Here's how the part is built. I have some questions about the finished solid (model axes, mm). Give positions to 0.01 mm unless a question says otherwise; leave off trailing zeros. Loops run counter-clockwise (first coordinate to the right, second up) from the corner with the lowest first, then second, coordinate; pieces in that order, holes last.
Q1. Suppose I cut it at B-B (x = 0). List the corners of the cut face in (y, z) for me, and give its area (3 significant figures).
Q2. I need wall thicknesses on probe 1 along X at (y, z) = (1.1, 0); probe 2 along Z at (x, y) = (0, 1.65); probe 3 along Z at (x, y) = (0, 0.8). Which ranges of each line are inside material? Lowest first, please.
Q3. I'm going to push a flat-ended pin straight in: P1, Ø3, axis at x = -1, z = 0.5, coming from the -Y side. Where does the tip first touch, or does it pass through?
Q4. Suppose I cut it at A-A (z = 0). List the corners of the cut face in (x, y) for me, and give its area (4 significant figures).
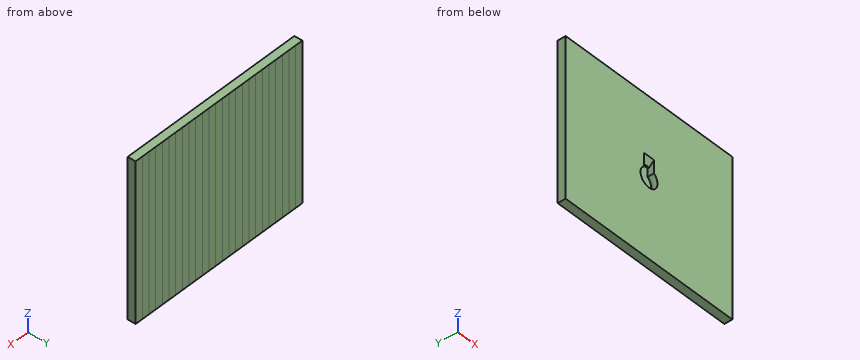
```python
from build123d import *

# Parameters (mm, degrees)
SKETCH1_W           = 59
SKETCH1_H           = 49.5
SKETCH1_R           = 3
BOSS_EXTRUDE1_DEPTH = 1.5
BOSS_EXTRUDE2_DEPTH = 49.5
CUT_EXTRUDE1_DEPTH  = 2
CUT_EXTRUDE3_DEPTH  = 65.105869466
CHAMFER3_SIZE       = 1.5
SKETCH7_W           = 59
SKETCH7_H           = 2.086537977
CUT_EXTRUDE5_DEPTH  = 58.762444547


with BuildPart() as part:
    # Sketch1 → Boss-Extrude1 (new body)
    with BuildSketch(Plane(origin=(0, 0, 0), x_dir=(1, 0, 0), z_dir=(0, 1, 0))):
        Rectangle(SKETCH1_W, SKETCH1_H)
        with Locations(Location((0, 0, 0), (0, 0, 270))):
            Circle(SKETCH1_R, mode=Mode.SUBTRACT)
    extrude(amount=BOSS_EXTRUDE1_DEPTH)

    # Sketch2 → Boss-Extrude2 (add)
    with BuildSketch(Plane(origin=(0, 0, -24.75), x_dir=(-1, 0, 0), z_dir=(0, 0, -1))):
        Polygon((-29.5, 1.5), (29.5, 1.5), (29.5, 2.5), (28.32, 4), (27.14, 2.5), (25.96, 4), (24.78, 2.5), (23.6, 4), (22.42, 2.5), (21.24, 4), (20.06, 2.5), (18.88, 4), (17.7, 2.5), (16.52, 4), (15.34, 2.5), (14.16, 4), (12.98, 2.5), (11.8, 4), (10.62, 2.5), (9.44, 4), (8.26, 2.5), (7.08, 4), (5.9, 2.5), (4.72, 4), (3.54, 2.5), (2.36, 4), (1.18, 2.5), (0, 4), (-1.18, 2.5), (-2.36, 4), (-3.54, 2.5), (-4.72, 4), (-5.9, 2.5), (-7.08, 4), (-8.26, 2.5), (-9.44, 4), (-10.62, 2.5), (-11.8, 4), (-12.98, 2.5), (-14.16, 4), (-15.34, 2.5), (-16.52, 4), (-17.7, 2.5), (-18.88, 4), (-20.06, 2.5), (-21.24, 4), (-22.42, 2.5), (-23.6, 4), (-24.78, 2.5), (-25.96, 4), (-27.14, 2.5), (-28.32, 4), (-29.5, 2.5), align=None)
    extrude(amount=-BOSS_EXTRUDE2_DEPTH)

    # Sketch3 → Cut-Extrude1 (cut)
    with BuildSketch(Plane(origin=(0, 0, 0), x_dir=(-1, 0, 0), z_dir=(0, -1, 0))):
        with BuildLine():
            Line((-1.75, -2.436698586), (-1.75, -5))
            Line((-1.75, -5), (1.75, -5))
            Line((1.75, -5), (1.75, -2.436698586))
            ThreePointArc((1.75, -2.436698586), (0, 3), (-1.75, -2.436698586))
        make_face()
    extrude(amount=-CUT_EXTRUDE1_DEPTH, mode=Mode.SUBTRACT)

    # Sketch4 → Cut-Extrude3 (cut, through all)
    with BuildSketch(Plane(origin=(29.5, 0, 0), x_dir=(0, 0, -1), z_dir=(1, 0, 0))):
        with BuildLine():
            Line((-24, 4), (-24.75, 4))
            Line((-24.75, 4), (-24.75, 3.25))
            ThreePointArc((-24.75, 3.25), (-24.530330086, 3.780330086), (-24, 4))
        make_face()
    cut_extrude3 = extrude(amount=-CUT_EXTRUDE3_DEPTH, mode=Mode.SUBTRACT)

    # Mirror1: Cut-Extrude3 across plane
    add(cut_extrude3.mirror(Plane.XY), mode=Mode.SUBTRACT)

    # Chamfer3
    chamfer3_edges = [part.edges().sort_by_distance(p)[0] for p in [
        (0, 0, 5),
    ]]
    chamfer(chamfer3_edges, length=CHAMFER3_SIZE)

    # Sketch7 → Cut-Extrude5 (cut, through all)
    with BuildSketch(Plane.XY.offset(24.75)):
        with Locations((0, 3.543268988)):
            Rectangle(SKETCH7_W, SKETCH7_H)
    extrude(amount=-CUT_EXTRUDE5_DEPTH, mode=Mode.SUBTRACT)


solid = part.part
```
Solutions:
1. outline: (0, -24.75) - (2.5, -24.75) - (2.5, 24.75) - (0, 24.75) - (0, 6.5) - (1.5, 5) - (2, 5) - (2, -3) - (0, -3) - close
1. area: 107 mm2
2. probe 1: x = -29.5 to -3, 3 to 29.5
2. probe 2: z = -24.75 to -3, 5 to 24.75
2. probe 3: z = -24.75 to -3, 5.7 to 24.75
3. P1: stops at y = 2
4. outline: (-29.5, 0) - (-3, 0) - (-3, 2) - (3, 2) - (3, 0) - (29.5, 0) - (29.5, 2.5) - (-29.5, 2.5) - close
4. area: 135.5 mm2
